Autodesk Inventor part; units mm, degrees
ref_plane "YZ Plane" through (0, 0, 0) normal (1, 0, 0) x (0, 1, 0)
ref_plane "XZ Plane" through (0, 0, 0) normal (0, 1, 0) x (-1, 0, 0)
ref_plane "XY Plane" through (0, 0, 0) normal (0, 0, 1) x (1, 0, 0)
sketch "Sketch1" plane through (0, 0, 0) normal (1, 0, 0) x (0, 1, 0)
  line L0 (0, 0) -> (0, -36)
  line L1 (0, -36) -> (38, -36)
  line L2 (0, 0) -> (-4, 0)
  line L3 (-4, 0) -> (-4, -40)
  line L4 (-4, -40) -> (38, -40)
  line L5 (38, -40) -> (38, -36)
  line L6 (0, 0) -> (-4, 0)
  line L7 (-4, 0) -> (-4, 27)
  line L8 (-4, 27) -> (0, 27)
  line L9 (0, 27) -> (0, 0)
  line L10 (-4, 27) -> (38, 27)
  line L11 (38, 27) -> (38, 31)
  line L12 (38, 31) -> (-4, 31)
  line L13 (-4, 31) -> (-4, 27)
  dimension "d0" = 36
  dimension "d1" = 38
  dimension "d2" = 4
  dimension "d3" = 40
  dimension "d28" = 27
  dimension "d29" = 42
  dimension "d30" = 4
extrude "Extrusion1" add sketch "Sketch1" along normal blind 21 contours L0 L1 L5 L4 L3 L2
fillet "Fillet1" radius 10 2 edges at (21, 38, -38) (0, 38, -38)
sketch "Sketch2" plane through (0, 0, -36) normal (0, 0, 1) x (1, 0, 0)
  arc A0 (10, 38) -> (0, 28) centre (10, 28) ccw
  line L0 (0, 28) -> (21, 28)
  line L1 (0, 28) -> (0, 0)
  line L2 (0, 28) -> (10.5, 28)
  circle A1 centre (10.5, 28) radius 8
  circle A2 centre (10.5, 28) radius 6.5
  line L3 (4, 28) -> (2.5, 28)
  circle A3 centre (3.25, 28) radius 1.1
  line L4 (17, 28) -> (18.5, 28)
  circle A4 centre (17.75, 28) radius 1.1
  line L5 (10.5, 28) -> (10.5, 36)
  line L6 (10.5, 28) -> (10.5, 20)
  line L7 (10.5, 36) -> (10.5, 34.5)
  line L8 (10.5, 20) -> (10.5, 21.5)
  circle A5 centre (10.5, 35.25) radius 1.1
  circle A6 centre (10.5, 20.75) radius 1.1
  circle A7 centre (10.5, 28) radius 3
  dimension "d7" = 10.5
  dimension "d8" = 16
  dimension "d9" = 13
  dimension "d10" = 2.2
  dimension "d11" = 2.2
  dimension "d12" = 2.2
  dimension "d13" = 2.2
  dimension "d14" = 6
extrude "Extrusion2" cut sketch "Sketch2" against normal blind 21 contours A2 A3 A1 L0 | A2 A3 L0 | L0 A1 A3 A2 | L0 A3 A2 | A1 A3 L0 | L0 A3 A1 | A7 L5 L0 | L0 L6 A7 | A5 A1 L5 A2 | A2 L5 A5 | A6 L6 A2 | A2 L6 A1 A6 | A5 A1 | A1 A6 | L5 A7 L0 | L0 A7 L6 | L5 A1 A5 A2 | A2 A5 L5 | L6 A6 A2 | A2 A6 A1 L6 | A4 L0 A1 | A1 L0 A2 A4 | A4 A2 L0 A1 | A1 L0 A4 | A4 A2 L0 | L0 A2 A4
fillet "Fillet2" radius 3 1 edges at (10.5, 0, -36)
extrude "Extrusion4" add sketch "Sketch1" along normal up to surface (21 mm away) contours L2 L7 L8 L9 | L8 L13 L12 L11 L10
fillet "Fillet3" radius 10 2 edges at (0, 38, 29) (21, 38, 29)
fillet "Fillet4" radius 3 1 edges at (10.5, 0, 27)
sketch "Sketch4" plane through (11, 38, 27) normal (0, 0, -1) x (-1, 0, 0)
  line L0 (-10, -10) -> (0.5, -10)
  circle A0 centre (0.5, -10) radius 1.5
  point P0 (11, -38)
  dimension "d35" = 10.5
  dimension "d36" = 3
extrude "Extrusion5" cut sketch "Sketch4" against normal blind 10
sketch "Sketch5" plane through (0, 0, -33) normal (0, 1, 0) x (1, 0, 0)
  line L0 (0, -57) -> (0, -60)
  line L1 (0, -57) -> (0, -32)
  line L2 (0, 0) -> (0, -57)
  line L3 (0, -32) -> (5, -32)
  line L4 (21, 0) -> (21, -57)
  line L5 (5, -32) -> (16, -32)
  line L6 (5, -32) -> (16, -32)
  line L7 (16, -32) -> (16, -21)
  line L8 (16, -21) -> (5, -21)
  line L9 (5, -21) -> (5, -32)
  circle A0 centre (5, -21) radius 1.5
  circle A1 centre (16, -21) radius 1.5
  circle A2 centre (5, -32) radius 1.5
  circle A3 centre (16, -32) radius 1.5
  point P0 (0, -33)
  dimension "d40" = 25
  dimension "d41" = 5
  dimension "d42" = 11
  dimension "d43" = 11
  dimension "d44" = 11
  dimension "d45" = 3
  dimension "d46" = 3
  dimension "d47" = 3
  dimension "d48" = 3
extrude "Extrusion6" cut sketch "Sketch5" against normal blind 10 contours A2 L9 L3 | L3 L5 A2 | L9 A2 L5 | A0 L8 L9 | L9 L8 A0 | A3 L7 L5 | L5 L7 A3 | A1 L7 L8 | L8 L7 A1
properties part number "L1"
Here's how the part is built. I have some questions about the finished solid (model axes, mm). A direction names the side the tool comes from. Round coordinates to 2 decimals unless told otherwise and drop trailing zeros. Order: outer loops, then holes, each group sorted by start corner. A loop starts at its lowest first (then second) coordinate and runs counter-clockwise, first axis right, second up. Notation, with made-up numbers: M 1.25,78 L 44.25,78 A32 cw 44.25,117 Z; hole C 88.25,72.5 d5. An arc over 180 degrees is marked long. Use CSV: the item, a comma, the result in double quotes.
1) On a 3-axis mill with a long thin cutter (end or side, diameter ignored), from which of +Z, -Z, +X, -X, +Y, -Y can I reach the whole of each face in a straight line? I mean faces 4 (the cylindrical face through (18.15, 34.99, -37.97)), 5 (the flat face through (10, 16, -36)), 6 (the cylindrical face through (8.1, 26.2, -38)). Say none if no direction works.
Taken from the geometry:
face 4,"+Z, -Z, +X, +Y"
face 5,"+X, -X, +Y"
face 6,"-Z"
2) I want a section at B-B (y = 13). List the corners of the cut face in (x, z) for me.
Taken from the geometry:
outline,"M 0,-40 L 21,-40 L 21,-36 L 0,-36 Z; M 0,27 L 21,27 L 21,31 L 0,31 Z"
3) I'm going to push flat-ended pins straight in: P1, Ø3.5, axis at x = 5, z = -1, coming from the +Y side; P2, Ø5, axis at x = 10.5, y = 28, coming from the -Z side; P3, Ø10, axis at x = 4, z = -30.5, coming from the +Y side. Where does each tip first touch, or does it pass through?
Taken from the geometry:
P1,"y = 0"
P2,"z = 27"
P3,"y = 1.34"
4) If we mould it in two halves opening along Y, with no side actions, what happens to faces 1 (the cylindrical face through (14.5, -1.97, -1.07)), 2 (the cylindrical face through (16.9, 27.3, -38)), 3 (the cylindrical face through (3.01, 35.15, -37.97))? For each: pulls with the +Y half, pulls with the -Y half, needs draft (parallel to the pull), parting line crosses it, or undercut.
Taken from the geometry:
face 1,"needs draft"
face 2,"undercut"
face 3,"pulls with the +Y half"
5) I need wall thicknesses on line 1 along X through (y, z) = (28, -37); line 2 along Z through (x, y) = (16, -2.75); line 3 along Y through (x, z) = (10.5, -37.7). Which ranges of each line are inside material? Lowest first, please. Write a range as [from, to].
Taken from the geometry:
line 1,"[0, 2.15], [4.35, 7.5], [13.5, 16.65], [18.85, 21]"
line 2,"[-40, -13.5], [-10.5, -2.5], [0.5, 31]"
line 3,"[-4, 19.65], [21.85, 25], [31, 34.15], [36.35, 38]"
6) I want a section at A-A (z = -12). List the corners of the cut face in (x, y) for me, then the cut area to 3 significant figures.
Taken from the geometry:
outline,"M 0,-4 L 3.5,-4 L 3.5,0 L 0,0 Z; M 6.5,-4 L 14.5,-4 L 14.5,0 L 6.5,0 Z; M 17.5,-4 L 21,-4 L 21,0 L 17.5,0 Z"
area,"60.0 mm^2"
7) I want a section at C-C (y = 35.25). List the corners of the cut face in (x, z) for me, then the cut area to 3 significant figures.
Taken from the geometry:
outline,"M 3.11,-40 L 9.4,-40 L 9.4,-36 L 3.11,-36 Z; M 3.11,27 L 17.89,27 L 17.89,31 L 3.11,31 Z; M 11.6,-40 L 17.89,-40 L 17.89,-36 L 11.6,-36 Z"
area,"109 mm^2"
8) I want a section at D-D (y = 1.5). List the corners of the cut face in (x, z) for me.
Taken from the geometry:
outline,"M 0,-40 L 21,-40 L 21,-35.6 L 0,-35.6 Z; M 0,26.6 L 21,26.6 L 21,31 L 0,31 Z"
